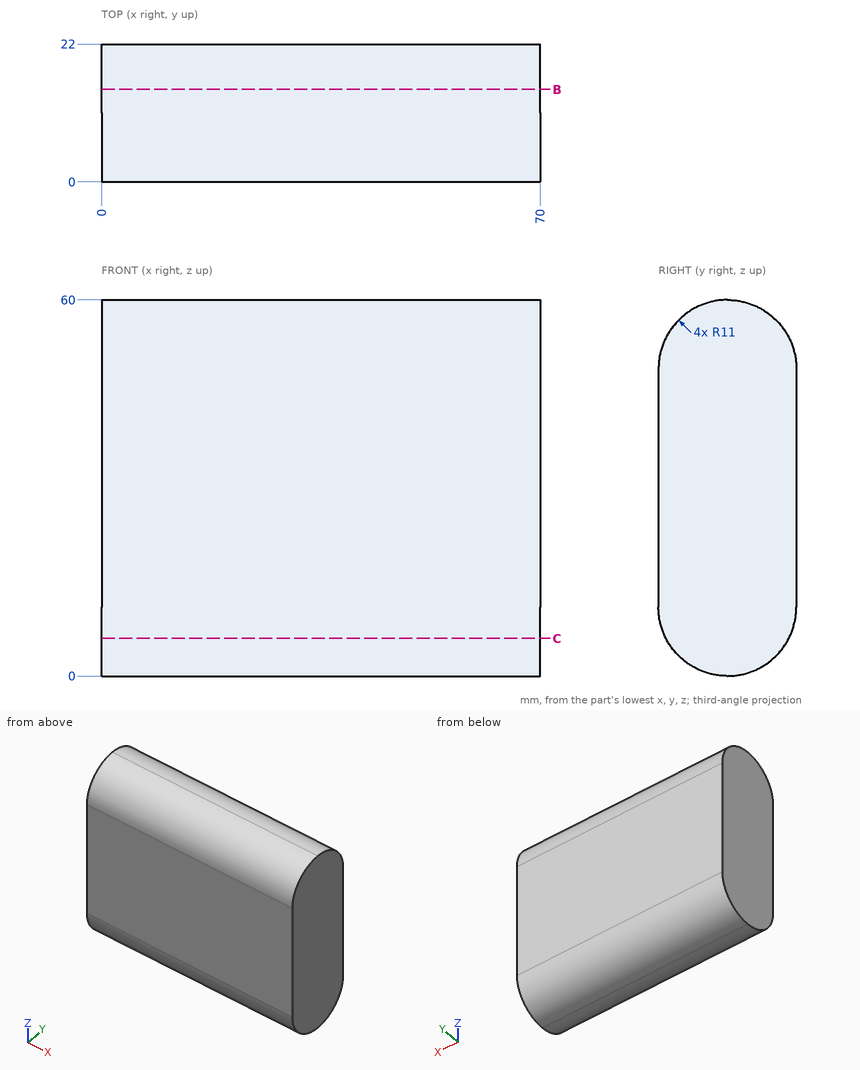
The drawing under review shows one solid part. Ordinate dimensions are in mm from its lowest x, y, z. Coordinates: 2 decimals unless noted, no trailing zeros. Order: outer loops, then holes, each group sorted by start corner. A loop starts at its lowest first (then second) coordinate and runs counter-clockwise, first axis right, second up. Notation, with made-up numbers: M 50.25,-27.75 L 88.25,-27.75 A26 cw 88.25,5.25 Z; hole C 36.25,-28.75 d6. An arc over 180 degrees is marked long. Use a Markdown table: item, result.
(1) Add section B-B (y = 14.75). Give the boundary of the cut face in (x, z), then the cut area to 3 significant figures.
Worked answers:
| item | result |
|---|---|
| outline | M 0,0.66 L 70,0.66 L 70,59.34 L 0,59.34 Z |
| area | 4,110 mm2 |
(2) Add section C-C (z = 6). Give the boundary of the cut face in (x, y).
Worked answers:
| item | result |
|---|---|
| outline | M 0,1.2 L 70,1.2 L 70,20.8 L 0,20.8 Z |
(3) For P1, Ø5, axis at x = 52.5, y = 15.5, coming from the +Z side; P2, Ø1, axis at y = 11.5, z = 54, coming from the -X side; P3, Ø5, axis at x = 31.5, y = 5, coming from the -Z side; P4, Ø1, axis at x = 23.5, z = 51.5, coming from the +Y side, all flat-tipped, find the tip position at first contact; note any pin that passes through.
Worked answers:
| item | result |
|---|---|
| P1 | stops at z = 59.82 |
| P2 | stops at x = 0 |
| P3 | stops at z = 0.57 |
| P4 | stops at y = 21.82 |
(4) Wall thickness on probe 1 along Y at (x, z) = (21.5, 49.5); probe 2 along Z at (x, y) = (50, 9.5); probe 3 along Z at (x, y) = (62, 18) (1 decimal): over which ranges is each line inside the solid? List them lowest first.
Worked answers:
| item | result |
|---|---|
| probe 1 | y = 0.01 to 21.99 |
| probe 2 | z = 0.1 to 59.9 |
| probe 3 | z = 2.5 to 57.5 |
